Model file for the job. Use its own axes, mm. A direction names the side the tool comes from. Round coordinates to 2 decimals unless told otherwise and drop trailing zeros. Order: outer loops, then holes, each group sorted by start corner. A loop starts at its lowest first (then second) coordinate and runs counter-clockwise, first axis right, second up. Notation, with made-up numbers: M 76.25,30.5 L 118.25,30.5 A18 cw 118.25,42.5 Z; hole C -16.5,-38.5 d7. An arc over 180 degrees is marked long. Return JSON: item names as keys, results as strings. Group by question number.
Item 1: Slice it at D-D on z = 16. Write the cut outline in (x, y), then the cut area to 3 significant figures.
Item 2: Pull direction Z, two halves, no side cores. Call faces 1 (the face through (0.493, -16.214, 0.325)), 2 (the face through (0.49, -19.99, 0.59)), 3 (the face through (0, -8, 0)): pulls with the +Z half, pulls with the -Z half, needs draft (parallel to the pull), parting line crosses it, or undercut.
Item 3: Slice it at B-B on z = 0. Write the cut outline in (x, y), then the cut area to 3 significant figures.
Item 4: Which spindle directions (+Z, -Z, +X, -X, +Y, -Y) get a long thin tool onto all of the face, cutting with end or side? Do faces 4 (the face through (1, -8, 0)), 5 (the face through (0.5, 3.2, 17.35)). Say none if no direction does.
Item 5: Slice it at C-C on x = 0.35. Write the cut outline in (y, z), then the cut area to 3 significant figures.
Item 6: Probe line 1 along Z through (x, y) = (0.35, -0.5); line 2 along Z through (x, y) = (0.4, -9.25); line 3 along Z through (x, y) = (0.8, -9.75). List the from-to ranges inside material, lowest first.
Item 7: Slice it at A-A on y = 0. Write the cut outline in (x, z), then the cut area to 3 significant figures.
Item 8: Pin check, flat tips, straight feed: pin 1 Ø0.5 at (x, y) = (0.5, 3) entering from -Z; pin 2 Ø8 at (y, z) = (2.5, -5) entering from +X; pin 3 Ø0.5 at (x, y) = (0.5, 5.5) entering from +Z. Stop position of each tip, or through.
from build123d import *

# Parameters (mm, degrees)
SKETCH1_R           = 20
SKETCH1_R_2         = 1.5
BOSS_EXTRUDE1_DEPTH = 1
SKETCH3_W           = 34.7
SKETCH3_H           = 20.778427125
CUT_EXTRUDE1_DEPTH  = 29.301943396


with BuildPart() as part:
    # Sketch1 → Boss-Extrude1 (new body)
    with BuildSketch(Plane(origin=(0, 0, 0), x_dir=(0, 0, -1), z_dir=(1, 0, 0))):
        Circle(SKETCH1_R)
        with Locations((0, 14.75)):
            Circle(SKETCH1_R_2, mode=Mode.SUBTRACT)
        with Locations((14.75, 0)):
            Circle(SKETCH1_R_2, mode=Mode.SUBTRACT)
        with Locations((0, -14.75)):
            Circle(SKETCH1_R_2, mode=Mode.SUBTRACT)
        with Locations((-14.75, 0)):
            Circle(SKETCH1_R_2, mode=Mode.SUBTRACT)
        with Locations((-8.485281374, 8.485281374)):
            Circle(SKETCH1_R_2, mode=Mode.SUBTRACT)
        with Locations((8.485281374, 8.485281374)):
            Circle(SKETCH1_R_2, mode=Mode.SUBTRACT)
        with Locations((8.485281374, -8.485281374)):
            Circle(SKETCH1_R_2, mode=Mode.SUBTRACT)
        with Locations((-8.485281374, -8.485281374)):
            Circle(SKETCH1_R_2, mode=Mode.SUBTRACT)
    extrude(amount=BOSS_EXTRUDE1_DEPTH)

    # Sketch3 → Cut-Extrude1 (cut, through all)
    with BuildSketch(Plane(origin=(1, 0, 0), x_dir=(0, 0, -1), z_dir=(1, 0, 0))):
        with Locations((0, 6.960786438)):
            Rectangle(SKETCH3_W, SKETCH3_H)
    extrude(amount=-CUT_EXTRUDE1_DEPTH, mode=Mode.SUBTRACT)


with BuildPart() as body_2:
    # of the pieces the cut leaves, the one that is kept (cut_extrude1_keep)
    add(part.part.solids().sort_by_distance((0, 9.948743639, 17.35))[0])


solid = body_2.part
Output values:
{
 "1": {"outline": "M 0,-12 L 1,-12 L 1,-3.43 L 0,-3.43 Z", "area": "8.57 mm²"},
 "2": {"face 1": "undercut", "face 2": "parting line crosses it", "face 3": "needs draft"},
 "3": {"outline": "M 0,-20 L 1,-20 L 1,-16.25 L 0,-16.25 Z; M 0,-13.25 L 1,-13.25 L 1,-3.43 L 0,-3.43 Z", "area": "13.6 mm²"},
 "4": {"face 4": "+Z, -Z, +X, +Y, -Y", "face 5": "+X, -X, +Y"},
 "5": {"outline": "M -3.43,-17.35 L -3.43,17.35 L 9.95,17.35 A20 ccw long 9.95,-17.35 Z; hole C -14.75,0 d3; hole C -8.49,-8.49 d3; hole C -8.49,8.49 d3", "area": "524 mm²"},
 "6": {"line 1": "-19.99 to -17.35, 17.35 to 19.99", "line 2": "-17.73 to -9.78, -7.19 to 7.19, 9.78 to 17.73", "line 3": "-17.46 to -9.29, -7.68 to 7.68, 9.29 to 17.46"},
 "7": {"outline": "M 0,-20 L 1,-20 L 1,-17.35 L 0,-17.35 Z; M 0,17.35 L 1,17.35 L 1,20 L 0,20 Z", "area": "5.30 mm²"},
 "8": {"pin 1": "z = -19.81", "pin 2": "through", "pin 3": "z = 19.3"}
}
